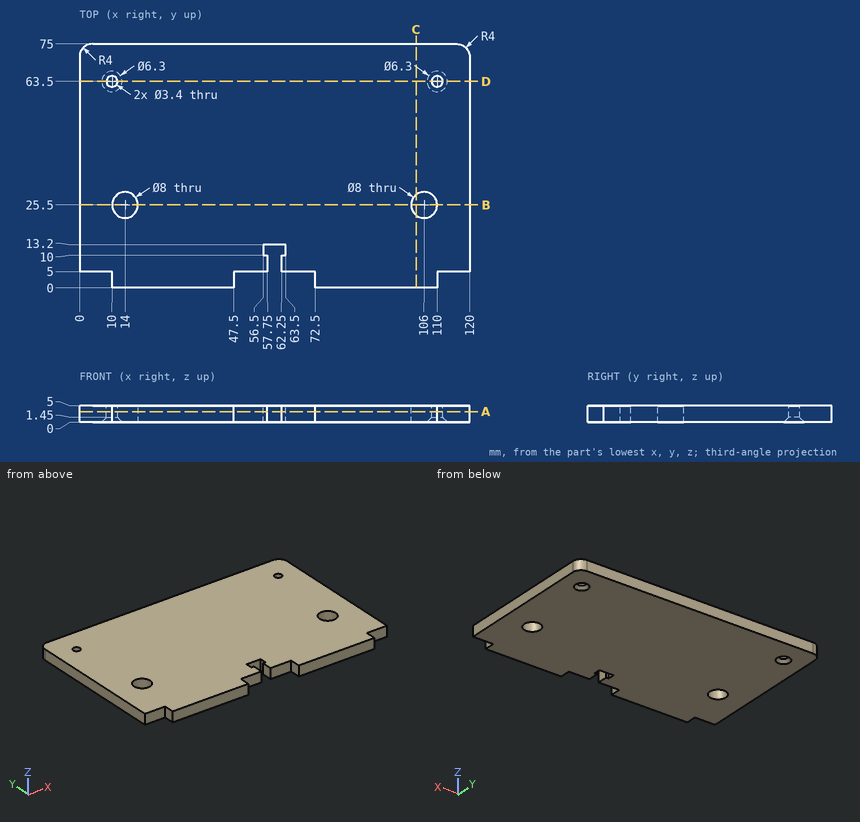
For this review, use the dimensioned drawing (mm, ordinates from the lowest corner) and the shaded views. Give positions to 0.01 mm unless a question says otherwise; leave off trailing zeros. Write each loop counter-clockwise with the first axis right and the second up, starting at its lowest first coordinate (ties: lowest second). Pieces come first, ordered by that corner, then holes. Notation, with made-up numbers: M -35,-10 L 20,-10 A14 cw 20,14 Z; hole C 11,89.25 d4. An arc over 180 degrees is marked long. Write item = value, one per line. Start each with the question number.
Q1. For line 1 (X direction, y = 25.5, z = 1.45); line 2 (Y direction, x = 106, z = 4); line 3 (Y direction, x = 10.5, z = 4.5), list the stretches that pass through material, from the lowest coordinate up.
Q2. Clearance check with flat-ended pins moving along their axes: pin 1 (2.5 mm diameter, centred on x = 50, z = 1.5, fed in from -Y); pin 2 (3 mm diameter, centred on x = 110, y = 63.5, fed in from +Z). State where each tip first meets the part, or that it passes through.
Q3. We need section B-B (y = 25.5). State the section outline as (x, z) points.
Q4. We need section D-D (y = 63.5). State the section outline as (x, z) points, plus the area to 3 significant figures.
Q5. We need section A-A (z = 3.2). State the section outline as (x, y) points.
Q6. We need section C-C (x = 103.5). State the section outline as (y, z) points.
Result set:
q1.line_1 = 0 to 10, 18 to 102, 110 to 120
q1.line_2 = 0 to 21.5, 29.5 to 75
q1.line_3 = 0 to 23.56, 27.44 to 61.88, 65.12 to 75
q2.pin_1 = 5
q2.pin_2 = through
q3.outline = M 0,0 L 10,0 L 10,5 L 0,5 Z; M 18,0 L 102,0 L 102,5 L 18,5 Z; M 110,0 L 120,0 L 120,5 L 110,5 Z
q4.outline = M 0,0 L 6.85,0 L 8.3,1.45 L 8.3,5 L 0,5 Z; M 11.7,1.45 L 13.15,0 L 106.85,0 L 108.3,1.45 L 108.3,5 L 11.7,5 Z; M 111.7,1.45 L 113.15,0 L 120,0 L 120,5 L 111.7,5 Z
q4.area = 562 mm2
q5.outline = M 0,5 L 10,5 L 10,0 L 47.5,0 L 47.5,5 L 57.75,5 L 57.75,10 L 56.5,10 L 56.5,13.2 L 63.5,13.2 L 63.5,10 L 62.25,10 L 62.25,5 L 72.5,5 L 72.5,0 L 110,0 L 110,5 L 120,5 L 120,71 A4 ccw 116,75 L 4,75 A4 ccw 0,71 Z; hole C 10,63.5 d3.4; hole C 14,25.5 d8; hole C 106,25.5 d8; hole C 110,63.5 d3.4
q6.outline = M 0,0 L 22.38,0 L 22.38,5 L 0,5 Z; M 28.62,0 L 75,0 L 75,5 L 28.62,5 Z
